Autodesk Inventor part; units mm, degrees
ref_plane "YZ Plane" through (0, 0, 0) normal (1, 0, 0) x (0, 1, 0)
ref_plane "XZ Plane" through (0, 0, 0) normal (0, 1, 0) x (-1, 0, 0)
ref_plane "XY Plane" through (0, 0, 0) normal (0, 0, 1) x (1, 0, 0)
sketch "Boceto1" plane through (0, 0, 0) normal (0, 1, 0) x (-1, 0, 0)
  circle A0 centre (0, 0) radius 79
  circle A1 centre (0, 0) radius 48
  dimension "d0" = 158
  dimension "d1" = 96
extrude "Extrusión1" add sketch "Boceto1" against normal blind 29
sketch "Boceto2" plane through (0, -29, 0) normal (0, -1, 0) x (1, 0, 0)
  circle A0 centre (0, 0) radius 56
  dimension "d4" = 112
extrude "Extrusión2" cut sketch "Boceto2" against normal blind 12
sketch "Boceto3" plane through (0, 0, 0) normal (0, 1, 0) x (1, 0, 0)
  circle A0 centre (0, 0) radius 64 construction
  circle A1 centre (0, 0) radius 48
  line L0 (0, 0) -> (64, 0) construction
  point P0 (32, 55.4256)
  point P1 (-32, 55.4256)
  point P2 (-64, 0)
  point P3 (-32, -55.4256)
  point P4 (32, -55.4256)
  dimension "d7" = 128
  dimension "d10" = 360
hole "Agujero1" at (64, 0, 0) at (32, 0, -55.4256) at (-32, 0, -55.4256) at (-64, 0, 0) at (-32, 0, 55.4256) at (32, 0, 55.4256) direction (0, -1, 0) diameter 10.106 depth 1.75
properties part number "4_AnilloComplementarioB"
Source: CAD feature listing. Evaluate the final solid. Frame: model axes, mm. A direction names the side the tool comes from. Round coordinates to 2 decimals unless told otherwise and drop trailing zeros. Loops run counter-clockwise (first coordinate to the right, second up) from the corner with the lowest first, then second, coordinate; pieces in that order, holes last.
(1) Section query A-A (x = 0). Output: boundary loops of the cut face in (y, z), and give its area (3 significant figures).
From the geometry:
outline: (-29, -79) - (0, -79) - (0, -48) - (-17, -48) - (-17, -56) - (-29, -56) - close; (-29, 56) - (-17, 56) - (-17, 48) - (0, 48) - (0, 79) - (-29, 79) - close
area: 1,610 mm2
(2) Material intervals for probe 1 along Z at (x, y) = (0, -24.25); probe 2 along Z at (x, y) = (0, -9); probe 3 along Z at (x, y) = (-32, -1.05), sorted ascending.
From the geometry:
probe 1: z = -79 to -56, 56 to 79
probe 2: z = -79 to -48, 48 to 79
probe 3: z = -72.23 to -60.48, -50.37 to -35.78, 35.78 to 50.37, 60.48 to 72.23
(3) Pull-direction query (X, two-part tool) for faces 1 (the cylindrical face through (58.23, -14.3, 53.39)), 2 (the flat face through (-16, -29, 54)), 3 (the flat face through (-32, -1.75, 55)), 4 (the cylindrical face through (58.99, -0.89, -0.66)); classes: +X half, -X half, draft (parallel to the pull), parting line (faces both ways), or undercut.
From the geometry:
face 1: parting line
face 2: draft
face 3: undercut
face 4: undercut
(4) Section query C-C (y = -5.75). Output: boundary loops of the cut face in (x, z).
From the geometry:
outline: circle Ø158 at (0, 0); hole circle Ø96 at (0, 0)
(5) Section query D-D (x = 64). Output: boundary loops of the cut face in (y, z).
From the geometry:
outline: (-29, -46.31) - (0, -46.31) - (0, -5.05) - (-1.75, -5.05) - (-1.75, 5.05) - (0, 5.05) - (0, 46.31) - (-29, 46.31) - close
(6) Section query B-B (z = 27). Output: boundary loops of the cut face in (x, y).
From the geometry:
outline: (-74.24, -29) - (-49.06, -29) - (-49.06, -17) - (-39.69, -17) - (-39.69, 0) - (-74.24, 0) - close; (39.69, -17) - (49.06, -17) - (49.06, -29) - (74.24, -29) - (74.24, 0) - (39.69, 0) - close
(7) Access query for faces 5 (the cylindrical face through (-69.01, -0.89, -0.66)), 6 (the cylindrical face through (51.73, -23.08, -21.45)), 7 (the flat face through (1, 0, -52)). Directions: +Z, -Z, +X, -X, +Y, -Y. A direction counts if a zero-diameter tool reaches every point of the face in a straight line with its end or side. Return the directions, or none.
From the geometry:
face 5: +Y
face 6: -Y
face 7: +Z, -Z, +X, -X, +Y
(8) Contact query for flat-ended pins moving along their axis: pin 1 Ø6 at (y, z) = (-14, -20) entering from -X; pin 2 Ø5 at (x, y) = (-49, -19) entering from -Z; pin 3 Ø3 at (x, z) = (-30.5, -56.5) entering from +Y; pin 4 Ø11 at (x, z) = (64.5, 0) entering from +Y. Output: stop coordinate, or through.
From the geometry:
pin 1: stops at x = -77.15
pin 2: stops at z = -63.87
pin 3: stops at y = -1.75
pin 4: stops at y = 0
